Autodesk Inventor part; units mm, degrees
ref_plane "YZ Plane" through (0, 0, 0) normal (1, 0, 0) x (0, 1, 0)
ref_plane "XZ Plane" through (0, 0, 0) normal (0, 1, 0) x (-1, 0, 0)
ref_plane "XY Plane" through (0, 0, 0) normal (0, 0, 1) x (1, 0, 0)
sketch "Sketch1" plane through (0, 0, 0) normal (0, 0, 1) x (1, 0, 0)
  circle A0 centre (19, 0) radius 4.65
  circle A1 centre (-6.5, -27) radius 4.65
  circle A2 centre (0, 0) radius 4.65
  circle A3 centre (25.5, -27) radius 4.65
  arc A4 (28.02, -35.95) -> (33.02, -30.95) centre (28.02, -30.95) ccw
  line L0 (33.02, 2.05) -> (33.02, -30.95)
  arc A5 (33.02, 2.05) -> (28.02, 7.05) centre (28.02, 2.05) ccw
  line L1 (-6.98, 7.05) -> (28.02, 7.05)
  arc A6 (-6.98, 7.05) -> (-11.98, 2.05) centre (-6.98, 2.05) ccw
  line L2 (-11.98, -30.95) -> (-11.98, 2.05)
  arc A7 (-11.98, -30.95) -> (-6.98, -35.95) centre (-6.98, -30.95) ccw
  line L3 (28.02, -35.95) -> (-6.98, -35.95)
  arc A8 (20.169, -15.05) -> (19.169, -16.05) centre (20.169, -16.05) ccw
  line L4 (20.169, -15.05) -> (21.169, -15.05)
  line L5 (21.169, -15.05) -> (21.169, -17.95)
  line L6 (21.169, -17.95) -> (20.169, -17.95)
  arc A9 (19.169, -16.95) -> (20.169, -17.95) centre (20.169, -16.95) ccw
  line L7 (19.169, -16.95) -> (19.169, -22.1)
  line L8 (19.169, -22.1) -> (-2.331, -22.1)
  line L9 (-2.331, -22.1) -> (-2.331, -10.9)
  line L10 (-2.331, -10.9) -> (19.169, -10.9)
  line L11 (19.169, -10.9) -> (19.169, -16.05)
  circle A10 centre (-6.48, -12.9) radius 2
  circle A11 centre (-3.844, -16.512) radius 0.75
  circle A12 centre (23.72, -20.1) radius 2
  line L12 (19.169, -16.05) -> (19.169, -16.95)
  circle A13 centre (25.5, -27) radius 3
  circle A14 centre (-6.5, -27) radius 3
  circle A15 centre (0, 0) radius 3
  circle A16 centre (19, 0) radius 3
  circle A17 centre (19, 0) radius 5
  dimension "d8" = 10
  dimension "d13" = 6
  dimension "d14" = 6
  dimension "d15" = 6
  dimension "d16" = 6
extrude "Extrusion1" add sketch "Sketch1" along normal blind 10 contours A0 | A1 | A2 | A3 | L3 A7 L2 A6 L1 A5 L0 A4 | L4 L5 L6 A9 L12 A8 | L12 L7 L8 L9 L10 L11 | A10 | A11 | A12 | A17
sketch "Sketch3" plane through (0, 0, 10) normal (0, 0, 1) x (1, 0, 0)
  line L0 (32.9618, -36.0107) -> (-11.98, 7.05)
  line L1 (-11.98, -35.95) -> (33.02, 7.05)
  circle A0 centre (8.9711, -16.071) radius 12.7
  circle A1 centre (-6.5, -27) radius 3
  circle A2 centre (19, 0) radius 3
  point P0 (0, 0)
  dimension "d2" = 25.4
  dimension "d17" = 2.2
extrude "Extrusion2" add sketch "Sketch3" along normal blind 17 contours A0 L1 L0 | L0 L1 A0 | L1 A0 L0 | L0 A0 L1
sketch "Sketch4" plane through (8.9711, -16.071, 27) normal (0, 0, 1) x (1, 0, 0)
  circle A0 centre (0, 0) radius 12.7
  circle A1 centre (0, 0) radius 7.5
  point P0 (-8.9711, 16.071)
  dimension "d5" = 15
extrude "Extrusion3" cut sketch "Sketch4" against normal through all contours A1
sketch "Sketch5" plane through (0, 0, 10) normal (0, 0, 1) x (1, 0, 0)
  circle A0 centre (19, 0) radius 3
  circle A1 centre (19, 0) radius 4.5
  circle A2 centre (0, 0) radius 4.5
  circle A3 centre (25.5, -27) radius 3
  circle A4 centre (25.5, -27) radius 4.5
  circle A5 centre (-6.5, -27) radius 3
  circle A6 centre (-6.5, -27) radius 4.5
  dimension "d9" = 9
  dimension "d10" = 9
  dimension "d18" = 9
  dimension "d19" = 9
extrude "Extrusion4" cut sketch "Sketch5" against normal blind 4
properties part number "Mount_DMD_KM100"
Build history of the part. All positions in model axes, mm. A direction names the side the tool comes from. Give positions to 0.01 mm unless a question says otherwise; leave off trailing zeros. Loops run counter-clockwise (first coordinate to the right, second up) from the corner with the lowest first, then second, coordinate; pieces in that order, holes last.
1) 3-axis set-ups, long thin cutter, end or side, ignore diameter. For faces 1 (the face through (15.2, -4.6, 10)), 2 (the face through (11, -35.95, 5)): which of +Z, -Z, +X, -X, +Y, -Y reach the whole face in a straight line?
Values follow:
face 1: +Z
face 2: +Z, -Z, +X, -X, -Y
2) Probe line 1 along Y through (x, z) = (25.5, 7.8); line 2 along Y through (x, z) = (25.5, 3.95); line 3 along X through (y, z) = (-2.5, 7.75). List the from-to ranges inside material, lowest first.
Values follow:
line 1: y = -35.95 to -31.5, -22.5 to 7.05
line 2: y = -35.95 to -30, -24 to 7.05
line 3: x = -11.98 to -3.74, 3.74 to 15.26, 22.74 to 33.02
3) Band-saw the part on D-D on y = -17.5. List the corners of the cut face in (x, z), then the cut area to 3 significant figures.
Values follow:
outline: (-11.98, 0) - (1.61, 0) - (1.61, 27) - (-3.65, 27) - (-3.65, 10) - (-11.98, 10) - close; (16.33, 0) - (33.02, 0) - (33.02, 10) - (21.59, 10) - (21.59, 27) - (16.33, 27) - close
area: 481 mm2
4) Band-saw the part on C-C on z = 2.25. List the corners of the cut face in (x, y).
Values follow:
outline: (-11.98, -30.95) arc R5 ccw to (-6.98, -35.95) - (28.02, -35.95) arc R5 ccw to (33.02, -30.95) - (33.02, 2.05) arc R5 ccw to (28.02, 7.05) - (-6.98, 7.05) arc R5 ccw to (-11.98, 2.05) - close; hole circle Ø6 at (-6.5, -27); hole circle Ø6 at (0, 0); hole circle Ø15 at (8.97, -16.07); hole circle Ø6 at (19, 0); hole circle Ø6 at (25.5, -27)
5) Band-saw the part on A-A on x = 25.5. List the corners of the cut face in (y, z), then the cut area to 3 significant figures.
Values follow:
outline: (-35.95, 0) - (-30, 0) - (-30, 6) - (-31.5, 6) - (-31.5, 10) - (-35.95, 10) - close; (-24, 0) - (7.05, 0) - (7.05, 10) - (-22.5, 10) - (-22.5, 6) - (-24, 6) - close
area: 358 mm2
6) Drop flat-ended pins along their axis: P1, Ø10, axis at x = -0.5, y = 1.5, coming from the +Z side; P2, Ø4, axis at x = 21.5, y = -19, coming from the -Z side; P3, Ø7, axis at x = 19, y = 0, coming from the +Z side; P4, Ø8, axis at y = -13, z = 14.5, coming from the +X side. Give the stop position or say it passes through.
Values follow:
P1: stops at z = 10
P2: stops at z = 0
P3: stops at z = 6
P4: stops at x = 21.67
7) Band-saw the part on B-B on y = 0. List the corners of the cut face in (x, z), then the cut area to 3 significant figures.
Values follow:
outline: (-11.98, 0) - (-3, 0) - (-3, 6) - (-4.5, 6) - (-4.5, 10) - (-11.98, 10) - close; (3, 0) - (16, 0) - (16, 6) - (14.5, 6) - (14.5, 10) - (4.5, 10) - (4.5, 6) - (3, 6) - close; (22, 0) - (33.02, 0) - (33.02, 10) - (23.5, 10) - (23.5, 6) - (22, 6) - close
area: 306 mm2
8) Two-plate mould, pull along Y, no slides. Class faces 3 (the face through (-10.6, 5.5, 4.9)), 4 (the face through (-8, -30, 6)), 5 (the face through (22.18, -23.96, 8.03)), 6 (the face through (14, -22, 27)): released by +Y, released by -Y, zero draft, split by the parting line, or undercut.
Values follow:
face 3: released by +Y
face 4: undercut
face 5: undercut
face 6: zero draft
